Print and shaded views of the part. All mm, measured from the part's lowest x, y and z. Give positions to 0.01 mm unless a question says otherwise; leave off trailing zeros. Loops run counter-clockwise (first coordinate to the right, second up) from the corner with the lowest first, then second, coordinate; pieces in that order, holes last.
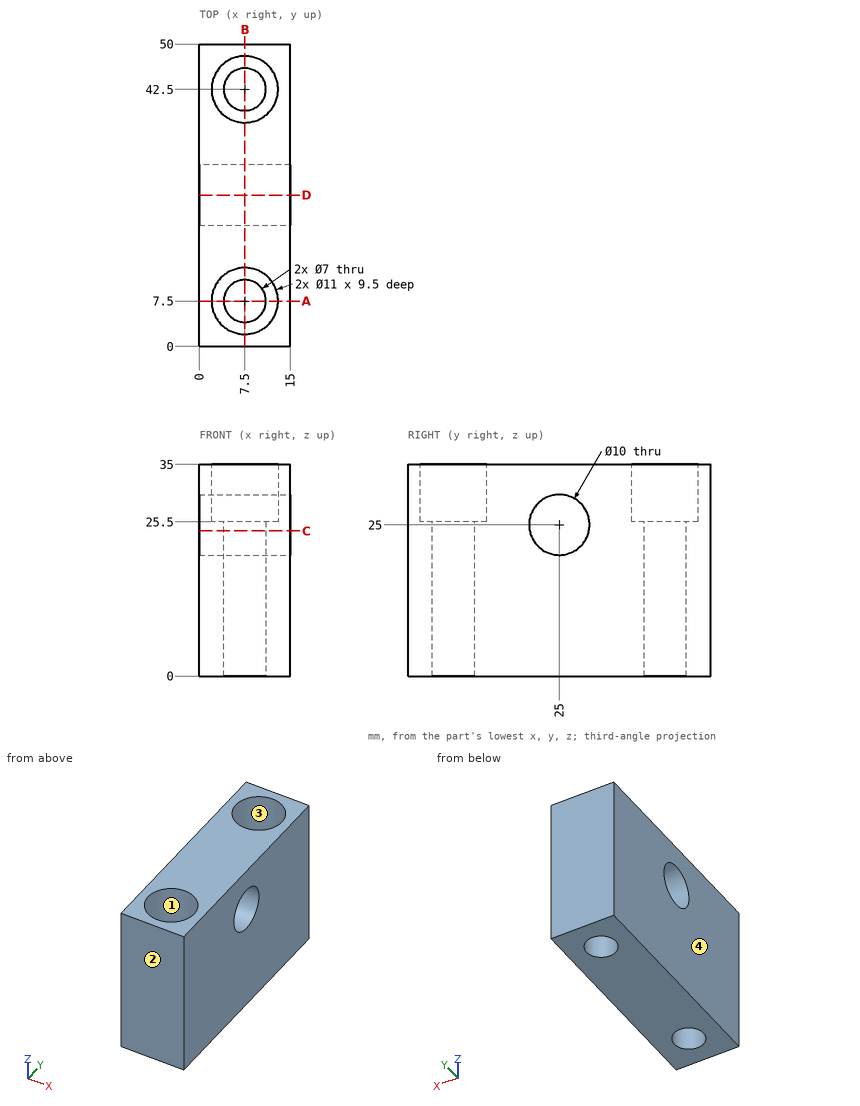
1. Pull direction Y, two halves, no side cores. Call the marked faces 1, 2, 3 and 4: released by +Y, released by -Y, zero draft, split by the parting line, or undercut.
Responses:
face 1: undercut
face 2: released by -Y
face 3: undercut
face 4: zero draft
2. Probe line 1 along Y through (x, z) = (7.5, 32.5); line 2 along Z through (x, y) = (4, 25); line 3 along Y through (x, z) = (7.5, 14.75). List the from-to ranges inside material, lowest first.
Responses:
line 1: y = 0 to 2, 13 to 37, 48 to 50
line 2: z = 0 to 20, 30 to 35
line 3: y = 0 to 4, 11 to 39, 46 to 50
3. Saw through at C-C, the plane z = 24. List the corners of the cut face in (x, y).
Responses:
outline: (0, 0) - (15, 0) - (15, 20.1) - (0, 20.1) - close; (0, 29.9) - (15, 29.9) - (15, 50) - (0, 50) - close; hole circle Ø7 at (7.5, 7.5); hole circle Ø7 at (7.5, 42.5)
4. Saw through at D-D, the plane y = 25. List the corners of the cut face in (x, z), and give its area (3 significant figures).
Responses:
outline: (0, 0) - (15, 0) - (15, 20) - (0, 20) - close; (0, 30) - (15, 30) - (15, 35) - (0, 35) - close
area: 375 mm2
5. Saw through at A-A, the plane y = 7.5. List the corners of the cut face in (x, z), and give its area (3 significant figures).
Responses:
outline: (0, 0) - (4, 0) - (4, 25.5) - (2, 25.5) - (2, 35) - (0, 35) - close; (11, 0) - (15, 0) - (15, 35) - (13, 35) - (13, 25.5) - (11, 25.5) - close
area: 242 mm2
6. Saw through at B-B, the plane x = 7.5. List the corners of the cut face in (y, z).
Responses:
outline: (0, 0) - (4, 0) - (4, 25.5) - (2, 25.5) - (2, 35) - (0, 35) - close; (11, 0) - (39, 0) - (39, 25.5) - (37, 25.5) - (37, 35) - (13, 35) - (13, 25.5) - (11, 25.5) - close; (46, 0) - (50, 0) - (50, 35) - (48, 35) - (48, 25.5) - (46, 25.5) - close; hole circle Ø10 at (25, 25)
